Build history of the part. All positions in model axes, mm. A direction names the side the tool comes from. Round coordinates to 2 decimals unless told otherwise and drop trailing zeros. Loops run counter-clockwise (first coordinate to the right, second up) from the corner with the lowest first, then second, coordinate; pieces in that order, holes last. Notation, with made-up numbers: M -14,86.5 L -6,86.5 A12 cw -6,103.5 Z; hole C -11.75,-1.75 d4. An arc over 180 degrees is marked long. One line per item, written item: value.
Autodesk Fusion 360 part; units mm, degrees
sketch "Sketch1" plane through (0, 0, 0) normal (0, 1, 0) x (1, 0, 0)
  line L0 (0, 0) -> (12.5, 0)
  line L1 (12.5, 0) -> (12.5, -12.1)
  line L2 (12.5, -12.1) -> (0, -12.1)
  line L3 (0, -12.1) -> (0, 0)
  line L4 (0, -12.1) -> (0, -14.6)
  line L5 (0, -14.6) -> (15, -14.6)
  line L6 (15, -14.6) -> (15, 0.0553)
  line L7 (15, 0.0553) -> (15, 2.5)
  line L8 (15, 2.5) -> (0, 2.5)
  line L9 (0, 2.5) -> (0, 0)
  dimension "d1" = 12.1
  dimension "d2" = 12.5
  dimension "d3" = 2.5
  dimension "d4" = 2.5
  dimension "d5" = 2.5
extrude "Extrude1" add sketch "Sketch1" along normal blind 11.1 contours L0 L1 L2 L3
extrude "Extrude3" add sketch "Sketch1" along normal blind -1.5 and the other way blind -2 contours L0 L1 L2 L4 L5 L6 L7 L8 L9
chamfer "Chamfer2" distance 2.461 angle 45 3 edges at (7.5, 2, 14.6) (15, 2, 6.05) (7.5, 2, -2.5)
Item 1: Slice it at C-C, the plane y = 10. Give the cut face in (x, z), and give its area (3 significant figures).
Check values:
outline: M 0,0 L 12.5,0 L 12.5,12.1 L 0,12.1 Z
area: 151 mm2
Item 2: Wall check: line 1 along Z through (x, y) = (6.5, 10.5); line 2 along X through (y, z) = (3, 2.5); line 3 along Y through (x, z) = (1.25, 10.5). Give the ranges that are in metal, low to high.
Check values:
line 1: z = 0 to 12.1
line 2: x = 0 to 12.5
line 3: y = 0 to 11.1
Item 3: Pull direction Z, two halves, no side cores. Call faces 1 (the face through (0, 5, 6)), 2 (the face through (6, 6, 12.1)), 3 (the face through (6, -1, 0)): pulls with the +Z half, pulls with the -Z half, needs draft (parallel to the pull), parting line crosses it, or undercut.
Check values:
face 1: needs draft
face 2: pulls with the +Z half
face 3: undercut
Item 4: Which spindle directions (+Z, -Z, +X, -X, +Y, -Y) get a long thin tool onto all of the face, cutting with end or side? Do faces 4 (the face through (12.5, 6, 6)), 5 (the face through (6, -1, 12.1)), 6 (the face through (6, 6, 0)), 7 (the face through (7.6, 0.75, 13.39)), 8 (the face through (7, -1, 14.6)). Say none if no direction does.
Check values:
face 4: +Z, -Z, +X, +Y
face 5: -X, -Y
face 6: -Z, +X, -X, +Y
face 7: +Z, +X, -X, +Y
face 8: +Z, +X, -X, +Y, -Y
Item 5: Slice it at D-D, the plane x = 13.25. Give the cut face in (y, z).
Check values:
outline: M -1.5,-2.5 L -0.46,-2.5 L 1.29,-0.75 L 1.29,12.85 L -0.46,14.6 L -1.5,14.6 Z
Item 6: Drop flat-ended pins along their axis: P1, Ø1, axis at y = 0.5, z = 5.5, coming from the +X side; P2, Ø3.5, axis at x = 8.5, z = 7, coming from the -Y side; P3, Ø2.5, axis at x = 8, y = 8, coming from the -Z side. Give the stop position or say it passes through.
Check values:
P1: stops at x = 14.54
P2: stops at y = 0
P3: stops at z = 0
